Autodesk Inventor part; units mm, degrees
ref_plane "YZ Plane" through (0, 0, 0) normal (1, 0, 0) x (0, 1, 0)
ref_plane "XZ Plane" through (0, 0, 0) normal (0, 1, 0) x (-1, 0, 0)
ref_plane "XY Plane" through (0, 0, 0) normal (0, 0, 1) x (1, 0, 0)
sketch "Sketch1" plane through (0, 0, 0) normal (0, 0, 1) x (1, 0, 0)
  arc A0 (0.75, -30.1532) -> (-0.75, -30.1532) centre (0, 0) ccw
  arc A1 (2.75, -32.0447) -> (-2.75, -32.0447) centre (0, 0) ccw
  line L0 (-0.75, -30.1532) -> (-0.75, -43.4447)
  line L1 (-0.75, -43.4447) -> (-2.75, -43.4447)
  line L2 (-2.75, -43.4447) -> (-2.75, -32.0447)
  line L3 (0.75, -30.1532) -> (0.75, -43.4447)
  line L4 (0.75, -43.4447) -> (2.75, -43.4447)
  line L5 (2.75, -43.4447) -> (2.75, -32.0447)
  dimension "d0" = 60.325
  dimension "d2" = 2
  dimension "d3" = 2
  dimension "d4" = 1.5
  dimension "d5" = 11.4
extrude "Extrusion1" add sketch "Sketch1" along normal blind 11.2
sketch "Sketch2" plane through (2.75, -43.4447, 0) normal (1, 0, 0) x (0, 0, -1)
  line L0 (0, 11.4) -> (-11.2, 11.4)
  line L1 (-11.2, 0) -> (-11.2, 11.4)
  circle A0 centre (-5.6, 5.7) radius 1.6
  point P0 (0, 43.4447)
  point P1 (-5.6, 11.4)
  point P2 (-11.2, 5.7)
  dimension "d8" = 3.2
extrude "Extrusion2" cut sketch "Sketch2" against normal through all
sketch "Sketch3" plane through (0, 0, 0) normal (0, 0, -1) x (-1, 0, 0)
  arc A0 (0.75, -30.1532) -> (-0.75, -30.1532) centre (0, 0) ccw
  line L0 (0.75, -43.4447) -> (0.75, -30.1532)
  line L1 (2.75, -43.4447) -> (0.75, -43.4447)
  line L2 (2.75, -32.0447) -> (2.75, -43.4447)
  arc A1 (2.75, -32.0447) -> (-2.75, -32.0447) centre (0, 0) ccw
  line L3 (-2.75, -43.4447) -> (-2.75, -32.0447)
  line L4 (-0.75, -43.4447) -> (-2.75, -43.4447)
  line L5 (-0.75, -30.1532) -> (-0.75, -43.4447)
extrude "Extrusion3" add sketch "Sketch3" along normal blind 2
sketch "Sketch4" plane through (0, 0, -2) normal (0, 0, -1) x (-1, 0, 0)
  line L0 (2.75, -43.4447) -> (2.75, -32.0447)
  arc A0 (2.75, -32.0447) -> (-2.75, -32.0447) centre (0, 0) ccw
  line L1 (-2.75, -32.0447) -> (-2.75, -43.4447)
  line L2 (2.75, -43.4447) -> (23.1319, -22.346)
  line L3 (-2.75, -43.4447) -> (-23.1319, -22.346)
extrude "Extrusion4" add sketch "Sketch4" against normal blind 2
fillet "Fillet1" radius 5.5 2 edges at (1.75, -43.4447, 11.2) (-1.75, -43.4447, 11.2)
fillet "Fillet2" radius 1 4 edges at (-0.75, -30.1532, 5.6) (-0.75, -30.1532, -1) (0.75, -30.1532, 5.6) (0.75, -30.1532, -1)
properties part number "CLAMP"
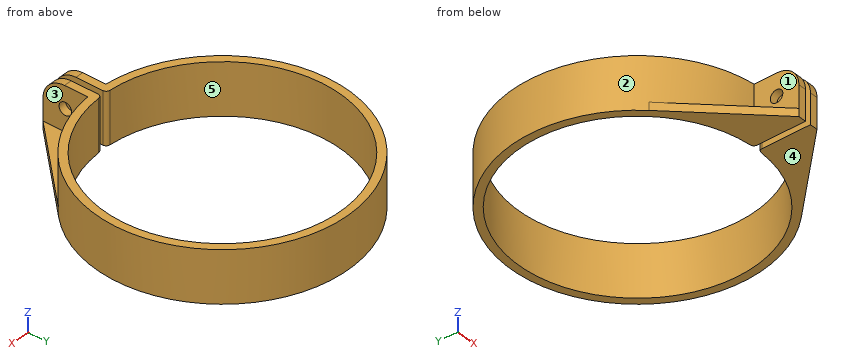
Here's how the part is built. I have some questions about the finished solid (model axes, mm). Face numbers are marked on the shaded views. A direction names the side the tool comes from. Round coordinates to 2 decimals unless told otherwise and drop trailing zeros. Loops run counter-clockwise (first coordinate to the right, second up) from the corner with the lowest first, then second, coordinate; pieces in that order, holes last. Notation, with made-up numbers: M 86.5,71 L 129.5,71 A18 ccw 129.5,79 Z; hole C 33.25,76.25 d4. An arc over 180 degrees is marked long. Write each question's results on one line, items separated by ' | '. Start each with the question number.
(1) I want a section at A-A (y = 0). Please give me the cut outline in (x, z), then the cut area to 3 significant figures.
(2) On a 3-axis mill with a long thin cutter (end or side, diameter ignored), from which of +Z, -Z, +X, -X, +Y, -Y can I reach the whole of each face in a straight line? I mean the marked faces 1, 2 and 3. Say none if no direction works.
(3) Will these pins go through, and if not, where does the flat tip stop? P1, Ø2, axis at y = 0, z = 0, coming from the +X side; P2, Ø1.5, axis at x = -12.5, z = 9, coming from the +Y side; P3, Ø6, axis at x = -15, z = 9, coming from the +Y side.
(4) If I drill on probe 1 along X at (y, z) = (-39.5, 7.25); probe 2 along X at (y, z) = (0, 7.25); probe 3 along Y at (x, z) = (2.1, 5.6), over which ranges is the centre line in solid material (lowest first)? Write a range as from..to.
(5) I want a section at D-D (y = -8). Please give me the cut outline in (x, z).
(6) I want a section at B-B (z = 1). Please give me the cut outline in (x, y).
(7) I want a section at C-C (x = -12). Please give me the cut outline in (y, z).
(8) Thinking about a two-plate mould opening in Z: for the marked faces 4 and 5, which applies, pulls with the +Z half, pulls with the -Z half, needs draft (parallel to the pull), parting line crosses it, or undercut?
Solved:
1) outline: M -32.16,-2 L -30.16,-2 L -30.16,11.2 L -32.16,11.2 Z; M 30.16,-2 L 32.16,-2 L 32.16,11.2 L 30.16,11.2 Z | area: 52.8 mm²
2) face 1: +Z, -X, -Y | face 2: +Z | face 3: +Z, +X, -Y
3) P1: stops at x = 32.16 | P2: stops at y = 29.94 | P3: stops at y = 29.84
4) probe 1: x = -2.75..-0.75, 0.75..2.75 | probe 2: x = -32.16..-30.16, 30.16..32.16 | probe 3: y = -43.44..-39.34, -36.14..-30.09, 30.09..32.09
5) outline: M -31.15,-2 L -29.08,-2 L -29.08,11.2 L -31.15,11.2 Z; M 29.08,-2 L 31.15,-2 L 31.15,11.2 L 29.08,11.2 Z
6) outline: M -2.75,-43.44 L -0.75,-43.44 L -0.75,-31.11 A1 ccw -1.69,-30.11 A30.16 cw long 1.69,-30.11 A1 ccw 0.75,-31.11 L 0.75,-43.44 L 2.75,-43.44 L 2.75,-32.04 A32.16 ccw long -2.75,-32.04 Z
7) outline: M -33.87,-2 L -27.67,-2 L -27.67,11.2 L -29.84,11.2 L -29.84,0 L -33.87,0 Z; M 27.67,-2 L 29.84,-2 L 29.84,11.2 L 27.67,11.2 Z
8) face 4: pulls with the -Z half | face 5: needs draft
